Check sheet for the modelled part. Datum: model origin and axes. Units: mm. Face numbers are marked on the shaded views. A direction names the side the tool comes from. Give positions to 0.01 mm unless a question says otherwise; leave off trailing zeros. Loops run counter-clockwise (first coordinate to the right, second up) from the corner with the lowest first, then second, coordinate; pieces in that order, holes last. Notation, with made-up numbers: (-29, 2.5) -> (16, 2.5) arc R18 ccw to (16, 27.5) -> close; hole circle Ø9 at (30.5, -23). An arc over 180 degrees is marked (long way). Write each question's results on one line, items separated by ' | '. Start each with the question number.
1. Material ranges on L1, parallel to Y at x = 21.5, z = -0.5; L2, parallel to X at y = 11, z = 5; L3, parallel to X at y = -3.25, z = 55, recorded low to high. Write a range as from..to.
2. Cross-section at A-A on x = -6. Record the boundary of the cut face in (y, z), and give its area (3 significant figures).
3. Gauge pin test, flat ends, axial feed: pin 1 Ø1.5 at (x, y) = (12, -5) entering from +Z; pin 2 Ø5 at (x, y) = (8, -12.5) entering from +Z; pin 3 Ø10.5 at (x, z) = (-14.24, 53.13) entering from -Y; pin 4 Ø17.5 at (x, z) = (-10.5, 51.5) entering from -Y. Record the tip position at first contact, or that the pin passes through.
4. Cross-section at C-C on z = 4. Record the boundary of the cut face in (x, y).
5. Mould release check, pull along Y, two halves, no side actions. Record for the marked faces 3, 4 and 5: +Y half, -Y half, draft (parallel to the pull), parting line (faces both ways), or undercut.
6. Tool access check on the marked faces 1 and 2. Record the directions out of +Z, -Z, +X, -X, +Y, -Y that give a thin tool (end or side, any length) a straight path to the whole face; none if there is none.
7. Cross-section at D-D on y = 12.5. Record the boundary of the cut face in (x, z).
8. Cross-section at B-B on y = -5. Record the boundary of the cut face in (x, z), and give its area (3 significant figures).
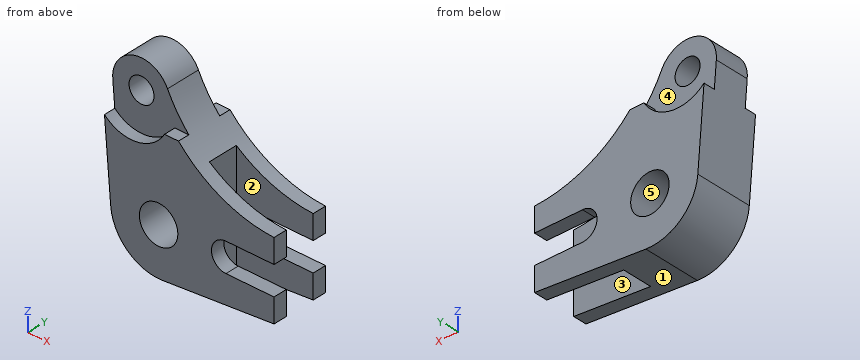
from build123d import *

# Parameters (mm, degrees)
SKETCH_R        = 10
SKETCH_R_2      = 6.5
PAD_DEPTH       = 15
SKETCH001_R     = 20
POCKET_DEPTH    = 6
SKETCH002_R     = 20
POCKET001_DEPTH = 6
SKETCH003_W     = 105.189392
SKETCH003_H     = 15.694074
POCKET002_DEPTH = 40
SKETCH004_W     = 18.945393
SKETCH004_H     = 8.112743
POCKET003_DEPTH = 6
SKETCH005_W     = 34.537269
SKETCH005_H     = 10.152644
POCKET004_DEPTH = 6


with BuildPart() as part:
    # Sketch → Pad (new body, symmetric)
    with BuildSketch(Plane.XZ):
        with BuildLine():
            ThreePointArc((-24.922099, -1.972055), (-16.174238, -19.062897), (2.11311, -24.910535))
            Line((2.11311, -24.910535), (60, -20))
            Line((60, -20), (60, -7.5))
            Line((60, -7.5), (35, -7.5))
            ThreePointArc((35, 7.5), (27.5, 0), (35, -7.5))
            Line((35, 7.5), (60, 7.5))
            Line((60, 7.5), (60, 20))
            ThreePointArc((-0.716595, 59.626032), (24.111636, 31.339626), (60, 20))
            ThreePointArc((-0.716595, 59.626032), (-18.14313, 67.607871), (-29.188307, 51.942687))
            Line((-24.922099, -1.972055), (-29.188307, 51.942687))
        make_face()
        Circle(SKETCH_R, mode=Mode.SUBTRACT)
        with Locations((-14.235047, 53.12592)):
            Circle(SKETCH_R_2, mode=Mode.SUBTRACT)
    extrude(amount=PAD_DEPTH, both=True)

    # Sketch001 → Pocket (cut)
    with BuildSketch(Plane.XZ.offset(15)):
        with Locations((-14.235047, 53.12592)):
            Circle(SKETCH001_R)
    extrude(amount=-POCKET_DEPTH, mode=Mode.SUBTRACT)

    # Sketch002 → Pocket001 (cut)
    with BuildSketch(Plane(origin=(0, 15, 0), x_dir=(1, 0, 0), z_dir=(0, 1, 0))):
        with Locations((-14.235047, -53.12592)):
            Circle(SKETCH002_R)
    extrude(amount=-POCKET001_DEPTH, mode=Mode.SUBTRACT)

    # Sketch003 → Pocket002 (cut)
    with BuildSketch(Plane(origin=(60, 0, 0), x_dir=(0, 0, 1), z_dir=(1, 0, 0))):
        with Locations((20.110367, 0)):
            Rectangle(SKETCH003_W, SKETCH003_H)
    extrude(amount=-POCKET002_DEPTH, mode=Mode.SUBTRACT)

    # Sketch004 → Pocket003 (cut)
    with BuildSketch(Plane.XZ.offset(15)):
        with Locations((5.87438, 47.182291)):
            Rectangle(SKETCH004_W, SKETCH004_H)
    extrude(amount=-POCKET003_DEPTH, mode=Mode.SUBTRACT)

    # Sketch005 → Pocket004 (cut)
    with BuildSketch(Plane(origin=(0, 15, 0), x_dir=(1, 0, 0), z_dir=(0, 1, 0))):
        with Locations((9.807045, -48.202242)):
            Rectangle(SKETCH005_W, SKETCH005_H)
    extrude(amount=-POCKET004_DEPTH, mode=Mode.SUBTRACT)


solid = part.part
Geometry says:
1) L1: -15..-7.85, 7.85..15 | L2: -25.47..-8.66, 8.66..29.41 | L3: -29.12..-20.46, -8.01..1.72
2) outline: (-15, -24.27) -> (15, -24.27) -> (15, -8) -> (-15, -8) -> close; (-15, 8) -> (15, 8) -> (15, 34.9) -> (9, 34.9) -> (9, 65.66) -> (-9, 65.66) -> (-9, 34.9) -> (-15, 34.9) -> close | area: 1,850 mm^2
3) pin 1: z = 42.14 | pin 2: z = 43.13 | pin 3: through | pin 4: y = -9
4) outline: (-25.39, -15) -> (-9.17, -15) -> (-9.17, 15) -> (-25.39, 15) -> close; (9.17, -15) -> (28.66, -15) -> (28.66, -7.85) -> (20, -7.85) -> (20, 7.85) -> (28.66, 7.85) -> (28.66, 15) -> (9.17, 15) -> close
5) face 3: undercut | face 4: +Y half | face 5: draft
6) face 1: -Z, +X, +Y, -Y | face 2: +Z, -Z, +X
7) outline: (-28.14, 38.76) -> (-24.92, -1.97) arc R25 ccw to (2.11, -24.91) -> (60, -20) -> (60, -7.5) -> (35, -7.5) arc R7.5 cw to (35, 7.5) -> (60, 7.5) -> (60, 20) arc R70 cw to (10.34, 43.13) -> (3.09, 43.13) arc R20 cw to start; hole circle Ø20 at (0, 0)
8) outline: (-29.19, 51.94) -> (-24.92, -1.97) arc R25 ccw to (2.11, -24.91) -> (20, -23.39) -> (20, 34.24) arc R70 cw to (-0.72, 59.63) arc R15 ccw to start; hole circle Ø13 at (-14.24, 53.13); hole circle Ø20 at (0, 0) | area: 3,210 mm^2
